from build123d import *

# Parameters (mm, degrees)
SCHIZZO1_R                   = 3.1
SCHIZZO1_R_2                 = 1.75
ESTRUSIONE_ESTRUSIONE1_DEPTH = 5


with BuildPart() as part:
    # Schizzo1 → Estrusione-Estrusione1 (new body)
    with BuildSketch(Plane.XY):
        with BuildLine():
            Line((0, 0), (0, 449))
            Line((0, 449), (171.5, 449))
            ThreePointArc((171.5, 449), (173.621320344, 448.121320344), (174.5, 446))
            Line((174.5, 446), (174.5, 417))
            ThreePointArc((174.5, 417), (177.428932188, 409.928932188), (184.5, 407))
            Line((184.5, 407), (264.5, 407))
            ThreePointArc((264.5, 407), (271.571067812, 409.928932188), (274.5, 417))
            Line((274.5, 417), (274.5, 446))
            ThreePointArc((274.5, 446), (275.378679656, 448.121320344), (277.5, 449))
            Line((277.5, 449), (331.145963874, 449))
            ThreePointArc((331.145963874, 449), (338.003609857, 446.278234097), (341.128274438, 439.594538314))
            Line((341.128274438, 439.594538314), (342.092482701, 423.405461686))
            ThreePointArc((342.092482701, 423.405461686), (345.217147282, 416.721765903), (352.074793265, 414))
            Line((352.074793265, 414), (375.181755612, 414))
            ThreePointArc((375.181755612, 414), (382.039401595, 416.721765903), (385.164066175, 423.405461686))
            Line((385.164066175, 423.405461686), (386.128274438, 439.594538314))
            ThreePointArc((386.128274438, 439.594538314), (389.252939019, 446.278234097), (396.110585002, 449))
            Line((396.110585002, 449), (449, 449))
            Line((449, 449), (449, 0))
            Line((449, 0), (0, 0))
        make_face()
        with Locations((11.5, 11.5)):
            Circle(SCHIZZO1_R, mode=Mode.SUBTRACT)
        with Locations((437.5, 11.5)):
            Circle(SCHIZZO1_R, mode=Mode.SUBTRACT)
        with Locations((437.5, 437.5)):
            Circle(SCHIZZO1_R, mode=Mode.SUBTRACT)
        with Locations((11.5, 437.5)):
            Circle(SCHIZZO1_R, mode=Mode.SUBTRACT)
        with Locations((309.5, 414)):
            Circle(SCHIZZO1_R_2, mode=Mode.SUBTRACT)
    extrude(amount=ESTRUSIONE_ESTRUSIONE1_DEPTH)


solid = part.part
Can you work these out from the model? Positions are in its coordinate system, mm. Give positions to 0.01 mm unless a question says otherwise; leave off trailing zeros. Loops run counter-clockwise (first coordinate to the right, second up) from the corner with the lowest first, then second, coordinate; pieces in that order, holes last. Notation, with made-up numbers: (7.5, -40) - (49.5, -40) arc R12 cw to (49.5, -33) - close; hole circle Ø5 at (70, 10.5). An arc over 180 degrees is marked (long way). Return JSON: item names as keys, results as strings.
1. I want a section at B-B on x = 220. Please give me the cut outline in (y, z).
Output values:
{"outline": "(0, 0) - (407, 0) - (407, 5) - (0, 5) - close"}
2. I'm going to push flat-ended pins straight in: pin 1 Ø1.5 at (x, z) = (177.5, 1) entering from +Y; pin 2 Ø7 at (x, y) = (437.5, 11.5) entering from +Z; pin 3 Ø3 at (x, y) = (309.5, 414) entering from +Z; pin 4 Ø2.5 at (x, z) = (359, 3.5) entering from +Y. Where does each tip first touch, or does it pass through?
Output values:
{"pin 1": "stops at y = 410.68", "pin 2": "stops at z = 5", "pin 3": "passes through", "pin 4": "stops at y = 414"}
3. If I drill on line 1 (Y direction, x = 11.5, z = 3.35); line 2 (Y direction, x = 376.5, z = 1.3); line 3 (Y direction, x = 201, z = 2.6), over which ranges is the centre line in solid material (lowest first)?
Output values:
{"line 1": "y = 0 to 8.4, 14.6 to 434.4, 440.6 to 449", "line 2": "y = 0 to 414.09", "line 3": "y = 0 to 407"}
4. We'd pull the mould along X, two halves only. Please class faces 1 (the face through (271.49, 409.85, 2.46)), 2 (the face through (177.35, 410.01, 2.46)), 3 (the face through (228, 228, 5)): +X half, -X half, draft (parallel to the pull), parting line (faces both ways), or undercut.
Output values:
{"face 1": "undercut", "face 2": "undercut", "face 3": "draft"}
5. I want a section at A-A on z = 1.2. Please give me the cut outline in (x, y), and give its area (3 significant figures).
Output values:
{"outline": "(0, 0) - (449, 0) - (449, 449) - (396.11, 449) arc R10 ccw to (386.13, 439.59) - (385.16, 423.41) arc R10 cw to (375.18, 414) - (352.07, 414) arc R10 cw to (342.09, 423.41) - (341.13, 439.59) arc R10 ccw to (331.15, 449) - (277.5, 449) arc R3 ccw to (274.5, 446) - (274.5, 417) arc R10 cw to (264.5, 407) - (184.5, 407) arc R10 cw to (174.5, 417) - (174.5, 446) arc R3 ccw to (171.5, 449) - (0, 449) - close; hole circle Ø6.2 at (11.5, 11.5); hole circle Ø6.2 at (11.5, 437.5); hole circle Ø3.5 at (309.5, 414); hole circle Ø6.2 at (437.5, 11.5); hole circle Ø6.2 at (437.5, 437.5)", "area": "196,000 mm²"}
